from build123d import *

# Parameters (mm, degrees)
SKETCH1_W           = 60
SKETCH1_H           = 140
BOSS_EXTRUDE1_DEPTH = 8
BOSS_EXTRUDE2_DEPTH = 60
CUT_EXTRUDE1_REACH  = 98.999
SKETCH5_R           = 4
SKETCH6_W           = 30
SKETCH6_H           = 30.146106113
CUT_EXTRUDE2_DEPTH  = 147.317421088
SKETCH7_R           = 3
CUT_EXTRUDE3_DEPTH  = 10


with BuildPart() as part:
    # Sketch1 → Boss-Extrude1 (new body)
    with BuildSketch(Plane(origin=(0, 0, 0), x_dir=(1, 0, 0), z_dir=(0, 1, 0))):
        Rectangle(SKETCH1_W, SKETCH1_H)
    extrude(amount=BOSS_EXTRUDE1_DEPTH)

    # Sketch3 → Boss-Extrude2 (add)
    with BuildSketch(Plane(origin=(30, 0, 0), x_dir=(0, 0, -1), z_dir=(1, 0, 0))):
        with BuildLine():
            Line((15, -15.146106113), (15, 0))
            Line((15, 0), (45, 0))
            Line((45, 0), (45, -15.146106113))
            ThreePointArc((45, -15.146106113), (30, -30.146106113), (15, -15.146106113))
        make_face()
    boss_extrude2 = extrude(amount=-BOSS_EXTRUDE2_DEPTH)

    # Mirror1: Boss-Extrude2 across plane
    add(boss_extrude2.mirror(Plane.XY))

    # Sketch5 → Cut-Extrude1 (cut, up to next)
    with BuildSketch(Plane(origin=(30, 0, 0), x_dir=(0, 0, -1), z_dir=(1, 0, 0)), mode=Mode.PRIVATE) as cut_extrude1_sk1:
        with Locations((30, -15.146106113)):
            Circle(SKETCH5_R)
    cut_extrude1_tool1 = extrude(cut_extrude1_sk1.sketch, amount=-CUT_EXTRUDE1_REACH, mode=Mode.PRIVATE) & part.part
    # Sketch5 → Cut-Extrude1 (cut, up to next)
    with BuildSketch(Plane(origin=(30, 0, 0), x_dir=(0, 0, -1), z_dir=(1, 0, 0)), mode=Mode.PRIVATE) as cut_extrude1_sk2:
        with Locations((-30, -15.146106113)):
            Circle(SKETCH5_R)
    cut_extrude1_tool2 = extrude(cut_extrude1_sk2.sketch, amount=-CUT_EXTRUDE1_REACH, mode=Mode.PRIVATE) & part.part
    add(cut_extrude1_tool1.solids().sort_by_distance((30, -15.146106, -30))[0], mode=Mode.SUBTRACT)
    add(cut_extrude1_tool2.solids().sort_by_distance((30, -15.146106, 30))[0], mode=Mode.SUBTRACT)

    # Sketch6 → Cut-Extrude2 (cut, through all)
    with BuildSketch(Plane.XY.offset(70)):
        with Locations((0, -15.073053057)):
            Rectangle(SKETCH6_W, SKETCH6_H)
    extrude(amount=-CUT_EXTRUDE2_DEPTH, mode=Mode.SUBTRACT)

    # Sketch7 → Cut-Extrude3 (cut)
    with BuildSketch(Plane.XZ):
        with Locations(Location((-16, -56, 0), (0, 0, 270))):
            Circle(SKETCH7_R)
        with Locations(Location((-16, 56, 0), (0, 0, 270))):
            Circle(SKETCH7_R)
        with Locations(Location((16, 56, 0), (0, 0, 270))):
            Circle(SKETCH7_R)
        with Locations(Location((16, -56, 0), (0, 0, 270))):
            Circle(SKETCH7_R)
    extrude(amount=-CUT_EXTRUDE3_DEPTH, mode=Mode.SUBTRACT)


solid = part.part
Geometry check sheet. Reference: the model listing, model coordinates, mm. A direction names the side the tool comes from. Round coordinates to 2 decimals unless told otherwise and drop trailing zeros. Order: outer loops, then holes, each group sorted by start corner. A loop starts at its lowest first (then second) coordinate and runs counter-clockwise, first axis right, second up. Notation, with made-up numbers: M 63,-2 L 78,-2 A33 ccw 78,37 Z; hole C -2.5,-28.5 d11. An arc over 180 degrees is marked long. Write each question's results on one line, items separated by ' | '. Start each with the question number.
1. Cross-section at D-D on z = -30. Record the boundary of the cut face in (x, y).
2. Set-up check for faces 4 (the face through (23, -7, 45)), 5 (the face through (23, -7, -45)), 6 (the face through (-15, -12, 27)): record each of +Z, -Z, +X, -X, +Y, -Y from which the full face is reachable in a straight line by a thin tool's end or side.
3. Material ranges on L1, parallel to X at y = 2.25, z = 56; L2, parallel to Z at x = 17, y = 6; L3, parallel to Y at x = -26, z = -30, recorded low to high. Write a range as from..to.
4. Cross-section at A-A on y = -3. Record the boundary of the cut face in (x, z).
5. Cross-section at B-B on z = -56. Record the boundary of the cut face in (x, y).
6. Go/stop test with flat-tipped pins: P1, Ø7, axis at y = -15.15, z = 30, coming from the -X side; P2, Ø1, axis at x = -21.5, y = -12.5, coming from the -Z side; P3, Ø9.5, axis at x = 16, z = 56, coming from the -Y side; P4, Ø12, axis at x = -9.5, y = -4.5, coming from the -Z side. Record where each tip stops, or that it passes through.
7. Draft check along X on faces 1 (the face through (-22, -7, 45)), 2 (the face through (-16, 4, 59)), 3 (the face through (30, 1, 1)). Enter one of: pulls with the +X half, pulls with the -X half, needs draft (parallel to the pull), parting line crosses it, or undercut.
8. Cross-section at C-C on x = 17.5. Record the boundary of the cut face in (y, z).
Resolved:
1) outline: M -30,-30.15 L -15,-30.15 L -15,-19.15 L -30,-19.15 Z; M -30,-11.15 L -15,-11.15 L -15,0 L 15,0 L 15,-11.15 L 30,-11.15 L 30,8 L -30,8 Z; M 15,-30.15 L 30,-30.15 L 30,-19.15 L 15,-19.15 Z
2) face 4: +Z, +X, -X, -Y | face 5: -Z, +X, -X, -Y | face 6: +Z, -Z, -Y
3) L1: -30..-19, -13..13, 19..30 | L2: -70..-58.83, -53.17..53.17, 58.83..70 | L3: -30.15..-19.15, -11.15..8
4) outline: M -30,-45 L -15,-45 L -15,-15 L -30,-15 Z; M -30,15 L -15,15 L -15,45 L -30,45 Z; M 15,-45 L 30,-45 L 30,-15 L 15,-15 Z; M 15,15 L 30,15 L 30,45 L 15,45 Z
5) outline: M -30,0 L -19,0 L -19,8 L -30,8 Z; M -13,0 L 13,0 L 13,8 L -13,8 Z; M 19,0 L 30,0 L 30,8 L 19,8 Z
6) P1: through | P2: z = -45 | P3: y = 0 | P4: z = -70
7) face 1: needs draft | face 2: undercut | face 3: pulls with the +X half
8) outline: M -15.15,-45 L 0,-45 L 0,-53.4 L 8,-53.4 L 8,53.4 L 0,53.4 L 0,45 L -15.15,45 A15 ccw -15.15,15 L 0,15 L 0,-15 L -15.15,-15 A15 ccw Z; M 0,-70 L 8,-70 L 8,-58.6 L 0,-58.6 Z; M 0,58.6 L 8,58.6 L 8,70 L 0,70 Z; hole C -15.15,-30 d8; hole C -15.15,30 d8
